Read the model definition and answer for the solid it produces. Units are mm, in the model's axes. Give positions to 0.01 mm unless a question says otherwise; leave off trailing zeros. Order: outer loops, then holes, each group sorted by start corner. A loop starts at its lowest first (then second) coordinate and runs counter-clockwise, first axis right, second up.
Item 1: Given pin 1 Ø1.2 at (x, y) = (81.5, 1.5) entering from -Z; pin 2 Ø2 at (y, z) = (2.5, -12) entering from -X; pin 3 Ø2 at (x, y) = (97.5, 1) entering from +Z, each flat-ended and moving along its own axis, determine where each tip first touches the part or whether it passes through.
Item 2: Find the intervals of material crossed by line 1 along Z through (x, y) = (142, 2.65); line 2 along X through (y, z) = (2.15, -31.5); line 3 along X through (y, z) = (0.9, 34.5), in increasing order.
Item 3: A cutting plane is placed at B-B (y = 2). State how many separate pieces and enclosed holes the cut face has, plus the area to 3 significant figures.
Item 4: A cutting plane is placed at C-C (x = -12). Write down the section's boundary in (y, z), plus the area to 3 significant figures.
Item 5: A cutting plane is placed at A-A (z = -22). Write down the section's boundary in (x, y), plus the area to 3 significant figures.
from build123d import *

# Parameters (mm, degrees)
SKETCH1_R           = 2
BOSS_EXTRUDE1_DEPTH = 4
SKETCH2_W           = 34
SKETCH2_H           = 4
SKETCH2_W_2         = 46
CUT_EXTRUDE1_DEPTH  = 151.792075389


with BuildPart() as part:
    # Sketch1 → Boss-Extrude1 (new body)
    with BuildSketch(Plane(origin=(0, 0, 0), x_dir=(1, 0, 0), z_dir=(0, 1, 0))):
        Polygon((146, -37.5), (-146, -37.5), (-146, 6.5), (-140, 6.5), (-140, 17.5), (-146, 17.5), (-146, 37.5), (-122.95, 37.5), (-122.95, 17.5), (-44, 17.5), (-44, 37.5), (44, 37.5), (44, 17.5), (122.95, 17.5), (122.95, 37.5), (146, 37.5), (146, 17.5), (140, 17.5), (140, 6.5), (146, 6.5), align=None)
        with Locations(Location((-142, 31.5, 0), (0, 0, 270))):
            Circle(SKETCH1_R, mode=Mode.SUBTRACT)
        with Locations(Location((142, 31.5, 0), (0, 0, 270))):
            Circle(SKETCH1_R, mode=Mode.SUBTRACT)
        with Locations(Location((0, 31.5, 0), (0, 0, 270))):
            Circle(SKETCH1_R, mode=Mode.SUBTRACT)
    extrude(amount=BOSS_EXTRUDE1_DEPTH)

    # Sketch2 → Cut-Extrude1 (cut, through all)
    with BuildSketch(Plane(origin=(0, 4, 0), x_dir=(1, 0, 0), z_dir=(0, 1, 0))):
        with Locations((95, -35.5)):
            Rectangle(SKETCH2_W, SKETCH2_H)
        with Locations((0, -35.5)):
            Rectangle(SKETCH2_W_2, SKETCH2_H)
        with Locations((-95, -35.5)):
            Rectangle(SKETCH2_W, SKETCH2_H)
    extrude(amount=-CUT_EXTRUDE1_DEPTH, mode=Mode.SUBTRACT)


solid = part.part
Response values:
1. pin 1: stops at z = -17.5
1. pin 2: stops at x = -140
1. pin 3: stops at z = 33.5
2. line 1: z = -37.5 to -33.5, -29.5 to -17.5, -6.5 to 37.5
2. line 2: x = -146 to -144, -140 to -122.95, -44 to -2, 2 to 44, 122.95 to 140, 144 to 146
2. line 3: x = -146 to -112, -78 to -23, 23 to 78, 112 to 146
3. separate pieces: 1
3. enclosed holes: 3
3. area: 18,100 mm2
4. outline: (0, -37.5) - (4, -37.5) - (4, 33.5) - (0, 33.5) - close
4. area: 284 mm2
5. outline: (-146, 0) - (-122.95, 0) - (-122.95, 4) - (-146, 4) - close; (-44, 0) - (44, 0) - (44, 4) - (-44, 4) - close; (122.95, 0) - (146, 0) - (146, 4) - (122.95, 4) - close
5. area: 536 mm2
